For this review, take the finished solid that the model builds, in its own axes (mm). A direction names the side the tool comes from. Round coordinates to 2 decimals unless told otherwise and drop trailing zeros. Order: outer loops, then holes, each group sorted by start corner. A loop starts at its lowest first (then second) coordinate and runs counter-clockwise, first axis right, second up. Notation, with made-up numbers: (9.25, 76) -> (21.25, 76) arc R9 ccw to (21.25, 90) -> close; hole circle Ø6 at (-0.5, 71). An arc over 180 degrees is marked (long way). Put each result on its own line as item: value. Start each with the question number.
```python
from build123d import *

# Parameters (mm, degrees)
SKETCH1_R           = 3.6
SKETCH1_R_2         = 3.5
SKETCH1_R_3         = 4.5
BOSS_EXTRUDE1_DEPTH = 3.14


with BuildPart() as part:
    # Sketch1 → Boss-Extrude1 (new body)
    # profile 1 of 10: a face of its own
    with BuildSketch(Plane.XY):
        with BuildLine():
            Line((38.651827519, 73.647136153), (-26.230787773, 73.647136153))
            Line((-26.230787773, 73.647136153), (-41.648963672, 73.647136153))
            add(Edge.make_bspline(
                [(-41.648963672, 73.647136153), (-44.643488897, 73.643488897), (-44.647136153, 70.648963672)],
                knots=[3.927599805, 3.927599805, 3.927599805, 5.497178156, 5.497178156, 5.497178156], degree=2, weights=[1, 0.707537269, 1]))
            Line((-44.647136153, 70.648963672), (-44.647136153, -70.648963672))
            add(Edge.make_bspline(
                [(-44.647136153, -70.648963672), (-44.643488897, -73.643488897), (-41.648963672, -73.647136153)],
                knots=[3.927599805, 3.927599805, 3.927599805, 5.497178156, 5.497178156, 5.497178156], degree=2, weights=[1, 0.707537269, 1]))
            Line((-41.648963672, -73.647136153), (27.093393639, -73.647136153))
            add(Edge.make_bspline(
                [(44.647136153, -54.550700861), (44.629350083, -55.622608831), (44.523578432, -56.687840097), (44.215717336, -58.366181711), (44.071515423, -58.983678353), (43.719242041, -60.213836545), (43.51280516, -60.820227412), (42.807525079, -62.600781834), (42.22206304, -63.742215888), (41.337337041, -65.108539745), (41.152542037, -65.37883334), (40.771685792, -65.906986664), (40.57512321, -66.165654002), (39.967232089, -66.92560473), (39.108255703, -67.89614606), (38.152323748, -68.781197278), (37.146406736, -69.622175477), (36.615243643, -70.022491506), (34.981146078, -71.128530207), (33.83112161, -71.747972893), (32.318701378, -72.376617626), (32.012437216, -72.49499434), (31.392225647, -72.716804064), (31.077608459, -72.820394039), (30.133341911, -73.105042114), (29.500121034, -73.261325902), (28.276366882, -73.499851982), (27.686391293, -73.587126278), (27.093393639, -73.647136153)],
                knots=[0.018260035, 0.018260035, 0.018260035, 0.018260035, 0.125, 0.125, 0.1875, 0.1875, 0.25, 0.25, 0.375, 0.375, 0.40625, 0.40625, 0.4375, 0.4375, 0.5, 0.5625, 0.5625, 0.625, 0.625, 0.75, 0.75, 0.78125, 0.78125, 0.8125, 0.8125, 0.875, 0.875, 0.932610516, 0.932610516, 0.932610516, 0.932610516], degree=3))
            Line((44.647136153, -54.550700861), (44.647136153, -53.896039233))
            Line((44.647136153, -53.896039233), (44.647136153, 22.020325098))
            ThreePointArc((44.647136153, 22.020325098), (42.730516554, 17.699527097), (39.139308268, 14.626100819))
            Line((39.139308268, 14.626100819), (39.139308268, 13.683084381))
            ThreePointArc((39.139308268, 13.683084381), (36.430045993, 7.142346655), (29.889308268, 4.433084381))
            Line((29.889308268, 4.433084381), (-36.027217939, 4.433084381))
            ThreePointArc((-36.027217939, 4.433084381), (-37.794984892, 5.165317428), (-38.527217939, 6.933084381))
            Line((-38.527217939, 6.933084381), (-38.527217939, 60.005147218))
            ThreePointArc((-38.527217939, 60.005147218), (-37.794984892, 61.772914171), (-36.027217939, 62.505147218))
            Line((-36.027217939, 62.505147218), (36.639308268, 62.505147218))
            ThreePointArc((36.639308268, 62.505147218), (38.40707522, 61.772914171), (39.139308268, 60.005147218))
            Line((39.139308268, 60.005147218), (39.139308268, 33.556674407))
            ThreePointArc((39.139308268, 33.556674407), (42.730516554, 30.483248128), (44.647136153, 26.162450128))
            Line((44.647136153, 26.162450128), (44.647136153, 67.670503394))
            Line((44.647136153, 67.670503394), (44.647136153, 70.648963672))
            add(Edge.make_bspline(
                [(44.647136153, 70.648963672), (44.643488897, 73.643488897), (41.648963672, 73.647136153)],
                knots=[3.927599805, 3.927599805, 3.927599805, 5.497178156, 5.497178156, 5.497178156], degree=2, weights=[1, 0.707537269, 1]))
            Line((41.648963672, 73.647136153), (38.651827519, 73.647136153))
        make_face()
        with BuildLine():
            ThreePointArc((-14.745996033, -51.265124074), (-17.044884469, -50.621435312), (-16.401195707, -48.322546875))
            Line((-16.401195707, -48.322546875), (-9.42859141, -44.400456958))
            ThreePointArc((-9.42859141, -44.400456958), (-7.129702973, -45.04414572), (-7.773391736, -47.343034157))
            Line((-7.773391736, -47.343034157), (-14.745996033, -51.265124074))
        make_face(mode=Mode.SUBTRACT)
        with Locations((-26.900831216, -26.517202566)):
            Circle(SKETCH1_R, mode=Mode.SUBTRACT)
        with BuildLine():
            ThreePointArc((1.254003967, -51.265124074), (-1.044884469, -50.621435312), (-0.401195707, -48.322546875))
            Line((-0.401195707, -48.322546875), (6.57140859, -44.400456958))
            ThreePointArc((6.57140859, -44.400456958), (8.870297027, -45.04414572), (8.226608264, -47.343034157))
            Line((8.226608264, -47.343034157), (1.254003967, -51.265124074))
        make_face(mode=Mode.SUBTRACT)
        with Locations((18.849494268, -29.546234455)):
            Circle(SKETCH1_R_2, mode=Mode.SUBTRACT)
        with Locations((32.960239, -21.476652312)):
            Circle(SKETCH1_R_2, mode=Mode.SUBTRACT)
    # profile 2 of 10: a face of its own
    with BuildSketch(Plane.XY):
        with BuildLine():
            add(Edge.make_bspline(
                [(-41.648963672, 73.647136153), (-44.643488897, 73.643488897), (-44.647136153, 70.648963672)],
                knots=[3.927599805, 3.927599805, 3.927599805, 5.497178156, 5.497178156, 5.497178156], degree=2, weights=[1, 0.707537269, 1]))
            Line((-41.648963672, 73.647136153), (-44.647136153, 73.647136153))
            Line((-44.647136153, 73.647136153), (-44.647136153, 70.648963672))
        make_face()
    # profile 3 of 10: a face of its own
    with BuildSketch(Plane.XY):
        with BuildLine():
            Line((44.647136153, 73.647136153), (41.648963672, 73.647136153))
            add(Edge.make_bspline(
                [(44.647136153, 70.648963672), (44.643488897, 73.643488897), (41.648963672, 73.647136153)],
                knots=[3.927599805, 3.927599805, 3.927599805, 5.497178156, 5.497178156, 5.497178156], degree=2, weights=[1, 0.707537269, 1]))
            Line((44.647136153, 70.648963672), (44.647136153, 73.647136153))
        make_face()
    # profile 4 of 10: a face of its own
    with BuildSketch(Plane.XY):
        with BuildLine():
            add(Edge.make_bspline(
                [(-44.647136153, -70.648963672), (-44.643488897, -73.643488897), (-41.648963672, -73.647136153)],
                knots=[3.927599805, 3.927599805, 3.927599805, 5.497178156, 5.497178156, 5.497178156], degree=2, weights=[1, 0.707537269, 1]))
            Line((-44.647136153, -70.648963672), (-44.647136153, -73.647136153))
            Line((-44.647136153, -73.647136153), (-41.648963672, -73.647136153))
        make_face()
    # profile 5 of 10: a face of its own
    with BuildSketch(Plane.XY):
        with BuildLine():
            Line((44.647136153, 22.020325098), (44.647136153, 26.162450128))
            ThreePointArc((44.647136153, 26.162450128), (42.730516554, 30.483248128), (39.139308268, 33.556674407))
            Line((39.139308268, 33.556674407), (39.139308268, 14.626100819))
            ThreePointArc((39.139308268, 14.626100819), (42.730516554, 17.699527097), (44.647136153, 22.020325098))
        make_face()
    # profile 6 of 10: a face of its own
    with BuildSketch(Plane.XY):
        with BuildLine():
            add(Edge.make_bspline(
                [(44.647136153, -54.550700861), (44.629350083, -55.622608831), (44.523578432, -56.687840097), (44.215717336, -58.366181711), (44.071515423, -58.983678353), (43.719242041, -60.213836545), (43.51280516, -60.820227412), (42.807525079, -62.600781834), (42.22206304, -63.742215888), (41.337337041, -65.108539745), (41.152542037, -65.37883334), (40.771685792, -65.906986664), (40.57512321, -66.165654002), (39.967232089, -66.92560473), (39.108255703, -67.89614606), (38.152323748, -68.781197278), (37.146406736, -69.622175477), (36.615243643, -70.022491506), (34.981146078, -71.128530207), (33.83112161, -71.747972893), (32.318701378, -72.376617626), (32.012437216, -72.49499434), (31.392225647, -72.716804064), (31.077608459, -72.820394039), (30.133341911, -73.105042114), (29.500121034, -73.261325902), (28.276366882, -73.499851982), (27.686391293, -73.587126278), (27.093393639, -73.647136153)],
                knots=[0.018260035, 0.018260035, 0.018260035, 0.018260035, 0.125, 0.125, 0.1875, 0.1875, 0.25, 0.25, 0.375, 0.375, 0.40625, 0.40625, 0.4375, 0.4375, 0.5, 0.5625, 0.5625, 0.625, 0.625, 0.75, 0.75, 0.78125, 0.78125, 0.8125, 0.8125, 0.875, 0.875, 0.932610516, 0.932610516, 0.932610516, 0.932610516], degree=3))
            Line((27.093393639, -73.647136153), (44.647136153, -73.647136153))
            Line((44.647136153, -73.647136153), (44.647136153, -54.550700861))
        make_face()
    # profile 7 of 10: a face of its own
    with BuildSketch(Plane.XY):
        with BuildLine():
            ThreePointArc((24.922228065, 29.508743732), (31.21939997, 34.382384037), (39.139308268, 33.556674407))
            Line((39.139308268, 33.556674407), (39.139308268, 60.005147218))
            ThreePointArc((39.139308268, 60.005147218), (38.40707522, 61.772914171), (36.639308268, 62.505147218))
            Line((36.639308268, 62.505147218), (-36.027217939, 62.505147218))
            ThreePointArc((-36.027217939, 62.505147218), (-37.794984892, 61.772914171), (-38.527217939, 60.005147218))
            Line((-38.527217939, 60.005147218), (-38.527217939, 6.933084381))
            ThreePointArc((-38.527217939, 6.933084381), (-37.794984892, 5.165317428), (-36.027217939, 4.433084381))
            Line((-36.027217939, 4.433084381), (29.889308268, 4.433084381))
            ThreePointArc((29.889308268, 4.433084381), (36.430045993, 7.142346655), (39.139308268, 13.683084381))
            Line((39.139308268, 13.683084381), (39.139308268, 14.626100819))
            ThreePointArc((39.139308268, 14.626100819), (31.21939997, 13.800391189), (24.922228065, 18.674031494))
            Line((24.922228065, 18.674031494), (24.922228065, 10.28797778))
            Line((24.922228065, 10.28797778), (-25.167870173, 10.28797778))
            Line((-25.167870173, 10.28797778), (-25.167870173, 56.21628744))
            Line((-25.167870173, 56.21628744), (24.922228065, 56.21628744))
            Line((24.922228065, 56.21628744), (24.922228065, 29.508743732))
        make_face()
        with Locations((-32.953932198, 40.341063425)):
            Circle(SKETCH1_R_3, mode=Mode.SUBTRACT)
    # profile 8 of 10: a face of its own
    with BuildSketch(Plane.XY):
        with BuildLine():
            Line((39.139308268, 14.626100819), (39.139308268, 33.556674407))
            ThreePointArc((39.139308268, 33.556674407), (31.21939997, 34.382384037), (24.922228065, 29.508743732))
            Line((24.922228065, 29.508743732), (24.922228065, 18.674031494))
            ThreePointArc((24.922228065, 18.674031494), (31.21939997, 13.800391189), (39.139308268, 14.626100819))
        make_face()
    # profile 9 of 10: a face of its own
    with BuildSketch(Plane.XY):
        with BuildLine():
            ThreePointArc((24.922228065, 18.674031494), (23.449484032, 24.091387613), (24.922228065, 29.508743732))
            Line((24.922228065, 29.508743732), (24.922228065, 56.21628744))
            Line((24.922228065, 56.21628744), (-25.167870173, 56.21628744))
            Line((-25.167870173, 56.21628744), (-25.167870173, 10.28797778))
            Line((-25.167870173, 10.28797778), (24.922228065, 10.28797778))
            Line((24.922228065, 10.28797778), (24.922228065, 18.674031494))
        make_face()
    # profile 10 of 10: a face of its own
    with BuildSketch(Plane.XY):
        with BuildLine():
            Line((24.922228065, 18.674031494), (24.922228065, 29.508743732))
            ThreePointArc((24.922228065, 29.508743732), (23.449484032, 24.091387613), (24.922228065, 18.674031494))
        make_face()
    extrude(amount=BOSS_EXTRUDE1_DEPTH)


solid = part.part
```
Item 1: Consider section C-C, the plane z = 1.25. Write out the cut boundary in (x, y), plus the area to 3 significant figures.
Item 2: Mouldability with a two-part tool opening along X and no side actions: class faces 1 (the face through (4.789, -49.277, 1.548)), 2 (the face through (44.647, -1, 2)), 3 (the face through (-1, -73.647, 2)), 4 (the face through (-33.54, 44.803, 1.548)) as +X half, -X half, draft (parallel to the pull), parting line (faces both ways), or undercut.
Item 3: For L1, parallel to X at y = -28.5, z = 2.4; L2, parallel to Y at x = 7.5, z = 0.3; L3, parallel to Y at x = 3, z = 2.75, list the stretches that pass through material, from the lowest coordinate up.
Item 4: Insertion check: pin 1 Ø4 at (x, y) = (32.96, -21.48) entering from +Z; pin 2 Ø1.5 at (x, y) = (10, 9) entering from -Z. Each pin has a flat end and moves straight along its axis. Give the tip position at first contact, or say it passes through.
Item 5: Consider section A-A, the plane y = 37.5. Write out the cut boundary in (x, z), plus the area to 3 significant figures.
Item 6: Consider section B-B, the plane x = 18. Write out the cut boundary in (y, z), plus the area to 3 significant figures.
Item 7: Tool access review of faces 5 (the face through (-1, 1, 0)), 6 (the face through (-11.211, -49.277, 1.548)): name each direction out of +Z, -Z, +X, -X, +Y, -Y from which nothing blocks a thin tool from reaching the whole face with its end or side.
Evaluation:
1. outline: (-44.65, -73.65) -> (44.65, -73.65) -> (44.65, 73.65) -> (-44.65, 73.65) -> close; hole circle Ø9 at (-32.95, 40.34); hole circle Ø7.2 at (-26.9, -26.52); hole (-16.4, -48.32) arc R1.69 ccw to (-14.75, -51.27) -> (-7.77, -47.34) arc R1.69 ccw to (-9.43, -44.4) -> close; hole (-0.4, -48.32) arc R1.69 ccw to (1.25, -51.27) -> (8.23, -47.34) arc R1.69 ccw to (6.57, -44.4) -> close; hole circle Ø7 at (18.85, -29.55); hole circle Ø7 at (32.96, -21.48)
1. area: 12,900 mm^2
2. face 1: undercut
2. face 2: +X half
2. face 3: draft
2. face 4: undercut
3. L1: x = -44.65 to -29.91, -23.9 to 15.51, 22.19 to 44.65
3. L2: y = -73.65 to -47.75, -44.19 to 73.65
3. L3: y = -73.65 to -50.28, -46.41 to 73.65
4. pin 1: passes through
4. pin 2: stops at z = 0
5. outline: (-44.65, 0) -> (-36.44, 0) -> (-36.44, 3.14) -> (-44.65, 3.14) -> close; (-29.46, 0) -> (44.65, 0) -> (44.65, 3.14) -> (-29.46, 3.14) -> close
5. area: 258 mm^2
6. outline: (-73.65, 0) -> (-32.94, 0) -> (-32.94, 3.14) -> (-73.65, 3.14) -> close; (-26.15, 0) -> (73.65, 0) -> (73.65, 3.14) -> (-26.15, 3.14) -> close
6. area: 441 mm^2
7. face 5: -Z, +X, -X, +Y, -Y
7. face 6: +Z, -Z
